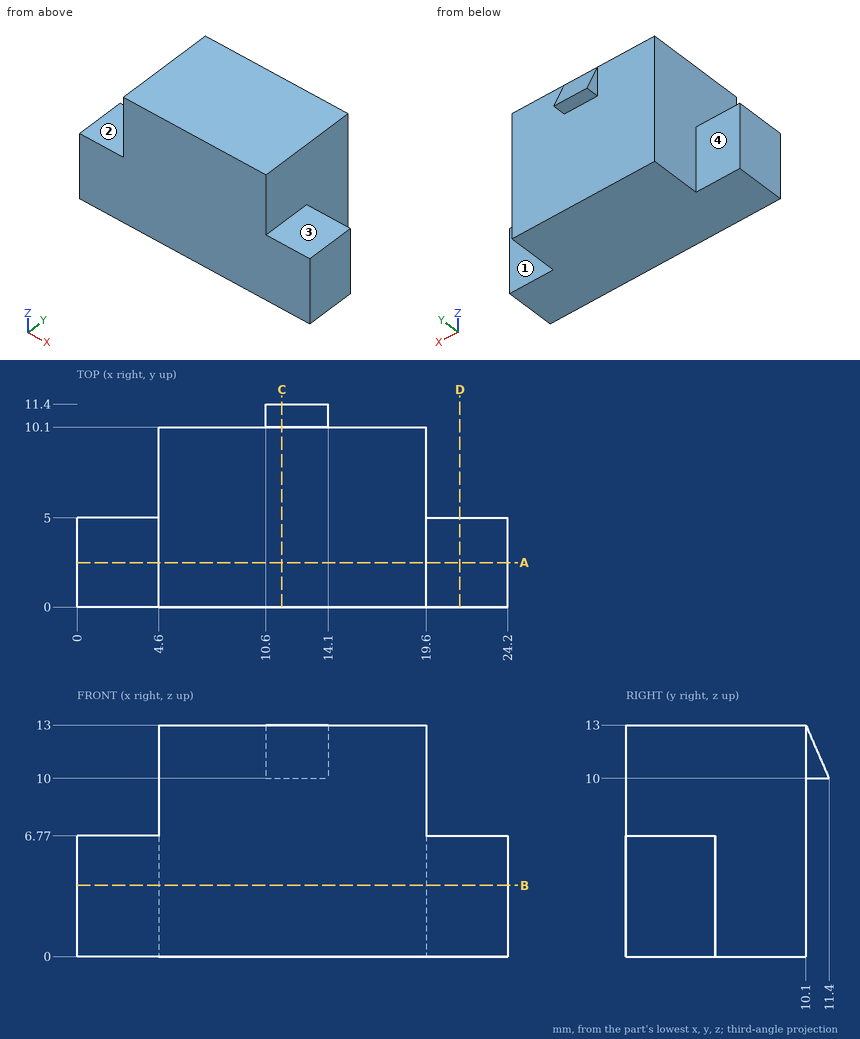
Can you work these out from the drawing? Everything is in mm from the part's minimum corner. A direction names the side the tool comes from. Coordinates: 2 decimals unless noted, no trailing zeros. Write each loop counter-clockwise with the first axis right and the second up, starting at its lowest first coordinate (ties: lowest second). Pieces come first, ordered by that corner, then holes. Notation, with made-up numbers: (29, 4) - (60, 4) arc R11 ccw to (60, 19) - close; hole circle Ø9 at (39.25, 42.5). An arc over 180 degrees is marked (long way). One line per item, written item: value.
1) Suppose I cut it at A-A on y = 2.5. Write out the boundary of the cut face in (x, z), and give its area (3 significant figures).
Model answer:
outline: (0, 0) - (24.2, 0) - (24.2, 6.77) - (19.6, 6.77) - (19.6, 13) - (4.6, 13) - (4.6, 6.77) - (0, 6.77) - close
area: 257 mm²
2) On a 3-axis mill with a long thin cutter (end or side, diameter ignored), from which of +Z, -Z, +X, -X, +Y, -Y can I reach the whole of each face in a straight line? I mean the marked faces 1, 2, 3 and 4. Say none if no direction works.
Model answer:
face 1: +Z, -Z, +X, +Y
face 2: +Z, -X, +Y, -Y
face 3: +Z, +X, +Y, -Y
face 4: +Z, -Z, -X, +Y
3) I need wall thicknesses on line 1 along Y through (x, z) = (13, 5); line 2 along X through (y, z) = (2.75, 11); line 3 along Y through (x, z) = (2.75, 1.25). Which ranges of each line are inside material? Lowest first, please.
Model answer:
line 1: y = 0 to 10.1
line 2: x = 4.6 to 19.6
line 3: y = 0 to 5
4) Suppose I cut it at D-D on x = 21.5. Write out the boundary of the cut face in (y, z), and give its area (4 significant figures).
Model answer:
outline: (0, 0) - (5, 0) - (5, 6.77) - (0, 6.77) - close
area: 33.85 mm²
5) Suppose I cut it at C-C on x = 11.5. Write out the boundary of the cut face in (y, z), and give its area (3 significant figures).
Model answer:
outline: (0, 0) - (10.1, 0) - (10.1, 10) - (11.4, 10) - (10.1, 13) - (0, 13) - close
area: 133 mm²
6) I'm going to push flat-ended pins straight in: P1, Ø1, axis at x = 12, y = 11, coming from the -Z side; P2, Ø3, axis at y = 4.5, z = 8.5, coming from the -X side; P3, Ø1.5, axis at x = 3, y = 2, coming from the +Z side. Where does each tip first touch, or does it pass through?
Model answer:
P1: stops at z = 10
P2: stops at x = 4.6
P3: stops at z = 6.77
7) Suppose I cut it at B-B on z = 4. Write out the boundary of the cut face in (x, y).
Model answer:
outline: (0, 0) - (24.2, 0) - (24.2, 5) - (19.6, 5) - (19.6, 10.1) - (4.6, 10.1) - (4.6, 5) - (0, 5) - close
